from build123d import *

# Parameters (mm, degrees)
F1_DEPTH = 50.8
F2_R     = 6.35
F3_DEPTH = 25.4


with BuildPart() as f1:
    # F0 (on Right) → F1 (new body)
    with BuildSketch(Plane.YZ):
        Polygon((42.91913, -27.839016), (42.91913, 22.960984), (30.21913, 22.960984), (30.21913, -15.374913), (-7.88087, -15.139016), (-7.88087, -27.839016), align=None)
    extrude(amount=F1_DEPTH)

    # F2 (on face) → F3 (cut)
    with BuildSketch(Plane.XZ.offset(-30.21913)):
        with Locations((23.75817, 0)):
            Circle(F2_R)
    extrude(amount=-F3_DEPTH, mode=Mode.SUBTRACT)


solid = f1.part
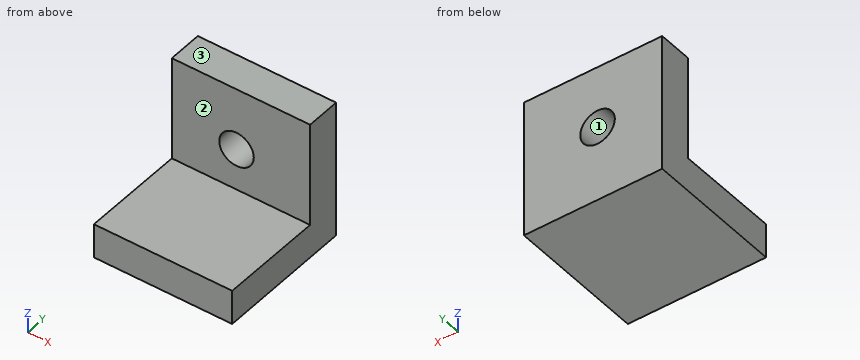
Source: CAD feature listing. Evaluate the final solid. Frame: model axes, mm. Face numbers are marked on the shaded views. Coordinates: 2 decimals unless noted, no trailing zeros. Write each loop counter-clockwise with the first axis right and the second up, starting at its lowest first coordinate (ties: lowest second). Pieces come first, ordered by that corner, then holes. Notation, with made-up numbers: M 65.25,42 L 97.25,42 A25 ccw 97.25,73 Z; hole C 37,-23 d4. An arc over 180 degrees is marked long. Use a Markdown table: item, result.
1) Mould query, pull axis Z, two halves, no side actions, for the marked faces 1, 2 and 3. Classes: pulls with the +Z half, pulls with the -Z half, needs draft (parallel to the pull), parting line crosses it, or undercut.
Conclusion:
| item | result |
|---|---|
| face 1 | undercut |
| face 2 | needs draft |
| face 3 | pulls with the +Z half |
2) Section B-B, the plane y = 32.5. Output: boundary loops of the cut face in (x, z), then the cut area to 3 significant figures.
Conclusion:
| item | result |
|---|---|
| outline | M 0,-27.84 L 50.8,-27.84 L 50.8,22.96 L 0,22.96 Z; hole C 23.76,0 d12.7 |
| area | 2,450 mm^2 |
3) Section A-A, the plane z = 0. Output: boundary loops of the cut face in (x, y).
Conclusion:
| item | result |
|---|---|
| outline | M 0,30.22 L 17.41,30.22 L 17.41,42.92 L 0,42.92 Z; M 30.11,30.22 L 50.8,30.22 L 50.8,42.92 L 30.11,42.92 Z |
4) Ray query, L1, parallel to Y at x = 42.5, z = 15.5; L2, parallel to Z at x = 7, y = 8; L3, parallel to Z at x = 29.5, y = 11. Return the intervals inside material, ascending.
Conclusion:
| item | result |
|---|---|
| L1 | y = 30.22 to 42.92 |
| L2 | z = -27.84 to -15.24 |
| L3 | z = -27.84 to -15.26 |
5) First-contact query: pin 1 Ø2 at (x, y) = (38.5, 29.5) entering from +Z; pin 2 Ø1.5 at (x, y) = (39, 19.5) entering from +Z; pin 3 Ø19 at (x, z) = (24.5, 3) entering from -Y. Flat tips, straight axial feed; report the tip coordinate or a pass-through.
Conclusion:
| item | result |
|---|---|
| pin 1 | stops at z = 22.96 |
| pin 2 | stops at z = -15.3 |
| pin 3 | stops at y = 30.22 |
6) Section D-D, the plane z = 17. Output: boundary loops of the cut face in (x, y).
Conclusion:
| item | result |
|---|---|
| outline | M 0,30.22 L 50.8,30.22 L 50.8,42.92 L 0,42.92 Z |
7) Section C-C, the plane x = 7.5. Output: boundary loops of the cut face in (y, z).
Conclusion:
| item | result |
|---|---|
| outline | M -7.88,-27.84 L 42.92,-27.84 L 42.92,22.96 L 30.22,22.96 L 30.22,-15.37 L -7.88,-15.14 Z |
